from build123d import *

# Parameters (mm, degrees)
SKETCH1_R           = 6
BOSS_EXTRUDE1_DEPTH = 10.8
FILLET1_R           = 1


with BuildPart() as part:
    # Sketch1 → Boss-Extrude1 (new body)
    with BuildSketch(Plane(origin=(0, 0, 0), x_dir=(1, 0, 0), z_dir=(0, 1, 0))):
        Polygon((9.741529803, 0), (6.888301783, 6.888301783), (0, 9.741529803), (-6.888301783, 6.888301783), (-9.741529803, 0), (-6.888301783, -6.888301783), (0, -9.741529803), (6.888301783, -6.888301783), align=None)
        with Locations(Location((0, 0, 0), (0, 0, 90))):
            Circle(SKETCH1_R, mode=Mode.SUBTRACT)
    extrude(amount=BOSS_EXTRUDE1_DEPTH)

    # Fillet1
    fillet1_edges = [part.edges().sort_by_distance(p)[0] for p in [
        (3.444150891, 10.8, -8.314915793),
        (8.314915793, 0, -3.444150891),
        (8.314915793, 0, 3.444150891),
        (-3.444150891, 10.8, -8.314915793),
        (-8.314915793, 10.8, -3.444150891),
        (-8.314915793, 10.8, 3.444150891),
        (-3.444150891, 10.8, 8.314915793),
        (3.444150891, 10.8, 8.314915793),
        (8.314915793, 10.8, 3.444150891),
        (8.314915793, 10.8, -3.444150891),
        (3.444150891, 0, 8.314915793),
        (-3.444150891, 0, 8.314915793),
        (-8.314915793, 0, 3.444150891),
        (-8.314915793, 0, -3.444150891),
        (-3.444150891, 0, -8.314915793),
        (3.444150891, 0, -8.314915793),
    ]]
    fillet(fillet1_edges, radius=FILLET1_R)


solid = part.part
Can you work these out from the model? Positions are in its coordinate system, mm. Round coordinates to 2 decimals unless told otherwise and drop trailing zeros. Loops run counter-clockwise (first coordinate to the right, second up) from the corner with the lowest first, then second, coordinate; pieces in that order, holes last. Notation, with made-up numbers: (41, 16.5) - (92, 16.5) arc R6 ccw to (92, 25.5) - close; hole circle Ø1 at (-37, 76). An arc over 180 degrees is marked (long way). Answer in a Markdown table with one row per item. Add a question column.
Q1. We'd pull the mould along X, two halves only. Please class faces 1 (the cylindrical face through (8.03, 10.5, -3.38)), 2 (the cylindrical face through (-3.29, 10.5, 8.07)), 3 (the cylindrical face through (-1.802, 5.324, -5.723)): pulls with the +X half, pulls with the -X half, needs draft (parallel to the pull), parting line crosses it, or undercut.
Q2. I need wall thicknesses on L1, parallel to X at y = 4, z = 0; L2, parallel to X at y = 4, z = -5; L3, parallel to Z at x = 2.75, y = 9.75. Which ranges of each line are inside material? Lowest first, please.
Q3. I want a section at A-A on y = 8. List the corners of the cut face in (x, z) for me, and give its area (3 significant figures).
A:
| question | item | result |
|---|---|---|
| 1 | face 1 | pulls with the +X half |
| 1 | face 2 | pulls with the -X half |
| 1 | face 3 | undercut |
| 2 | L1 | -9.74 to -6, 6 to 9.74 |
| 2 | L2 | -7.67 to -3.32, 3.32 to 7.67 |
| 2 | L3 | -8.6 to -5.33, 5.33 to 8.6 |
| 3 | outline | (-9.74, 0) - (-6.89, -6.89) - (0, -9.74) - (6.89, -6.89) - (9.74, 0) - (6.89, 6.89) - (0, 9.74) - (-6.89, 6.89) - close; hole circle Ø12 at (0, 0) |
| 3 | area | 155 mm^2 |
